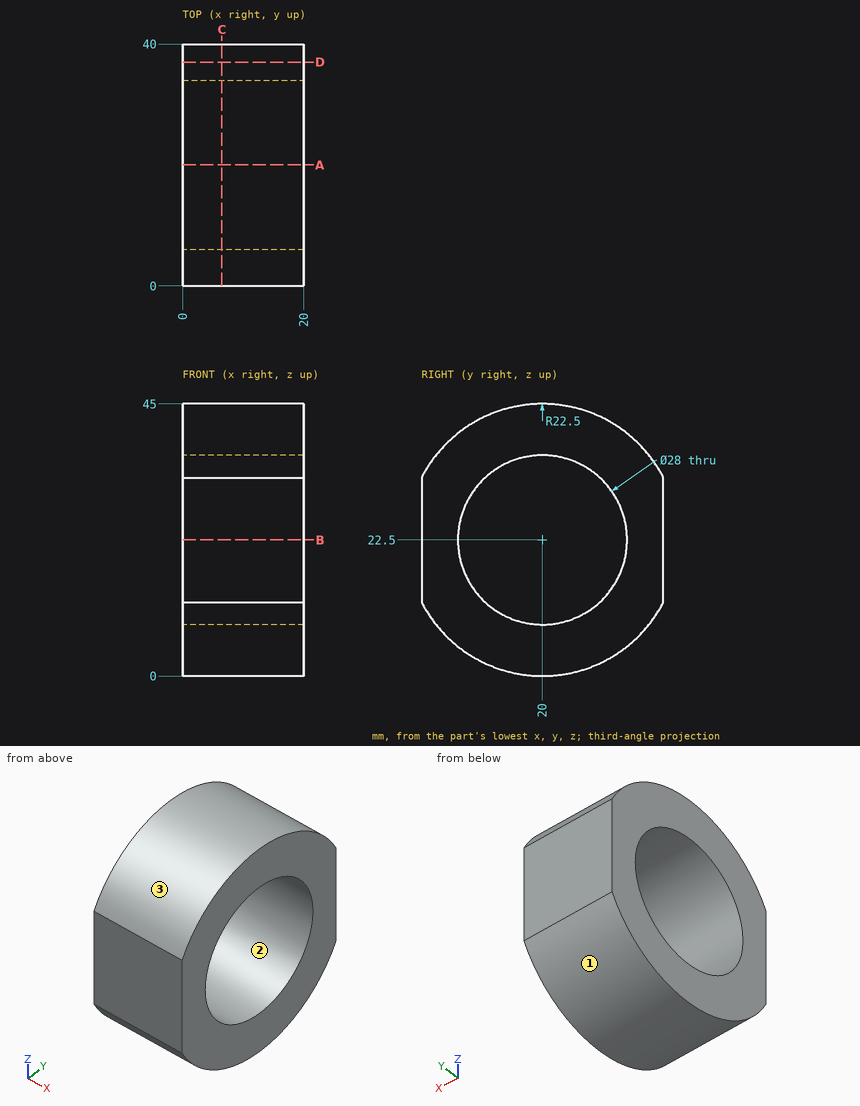
Input: dimensioned drawing with shaded views. Units: mm. Origin: part minimum x, y, z. Coordinates: 2 decimals unless noted, no trailing zeros. Loops run counter-clockwise (first coordinate to the right, second up) from the corner with the lowest first, then second, coordinate; pieces in that order, holes last. Notation, with made-up numbers: M 19,20 L 24,20 A17 ccw 24,52 Z; hole C 87,-39 d1. An arc over 180 degrees is marked long. Use a Markdown table: item, result. Add a question column.
Q1. Section query D-D, the plane y = 37. Return loops of the section in (x, z), and give its area (3 significant figures).
Q2. Material intervals for L1, parallel to Z at x = 7.5, y = 20; L2, parallel to Z at x = 12.25, y = 32; L3, parallel to Y at x = 18, z = 15.5, sorted ascending.
Q3. Section query B-B, the plane z = 22.5. Return loops of the section in (x, y).
Q4. Section query A-A, the plane y = 20. Return loops of the section in (x, z), and give its area (3 significant figures).
Q5. Draft query along Z for the marked faces 1, 2 and 3. Return one class per face: pulls with the +Z half, pulls with the -Z half, needs draft (parallel to the pull), parting line crosses it, or undercut.
Q6. Section query C-C, the plane x = 6.5. Return loops of the section in (y, z).
Q7. First-contact query: pin 1 (6 mm diameter, centred on x = 15, z = 6.5, fed in from -Y); pin 2 (8 mm diameter, centred on x = 8.5, y = 27.5, fed in from +Z); pin 3 (1.5 mm diameter, centred on x = 6, z = 37, fed in from +Y). Flat tips, straight axial feed; report the tip coordinate or a pass-through.
Result:
| question | item | result |
|---|---|---|
| 1 | outline | M 0,7.76 L 20,7.76 L 20,37.24 L 0,37.24 Z |
| 1 | area | 590 mm2 |
| 2 | L1 | z = 0 to 8.5, 36.5 to 45 |
| 2 | L2 | z = 3.47 to 15.29, 29.71 to 41.53 |
| 2 | L3 | y = 0 to 7.88, 32.12 to 40 |
| 3 | outline | M 0,0 L 20,0 L 20,6 L 0,6 Z; M 0,34 L 20,34 L 20,40 L 0,40 Z |
| 4 | outline | M 0,0 L 20,0 L 20,8.5 L 0,8.5 Z; M 0,36.5 L 20,36.5 L 20,45 L 0,45 Z |
| 4 | area | 340 mm2 |
| 5 | face 1 | pulls with the -Z half |
| 5 | face 2 | undercut |
| 5 | face 3 | pulls with the +Z half |
| 6 | outline | M 0,12.19 A22.5 ccw 40,12.19 L 40,32.81 A22.5 ccw 0,32.81 Z; hole C 20,22.5 d28 |
| 7 | pin 1 | stops at y = 1.64 |
| 7 | pin 2 | stops at z = 44.73 |
| 7 | pin 3 | stops at y = 37.81 |
